```python
from build123d import *

# Parameters (mm, degrees)
BOSS_EXTRUDE1_DEPTH            = 44
CUT_EXTRUDE1_REACH             = 129.516
SKETCH5_R                      = 23
CUT_EXTRUDE1_DIRECTION_2_REACH = 129.516
CUT_EXTRUDE2_REACH             = 137.133
SKETCH6_R                      = 5
CUT_EXTRUDE3_REACH             = 137.133
SKETCH7_R                      = 9.5


with BuildPart() as part:
    # Sketch1 → Boss-Extrude1 (new, symmetric)
    with BuildSketch(Plane(origin=(0, 0, 0), x_dir=(0, 0, -1), z_dir=(1, 0, 0))):
        with BuildLine():
            Line((0, 0), (0, -65))
            Line((0, -65), (12, -65))
            Line((12, -65), (12, -30))
            Line((12, -30), (75, -30))
            Line((75, -30), (75, -27))
            ThreePointArc((75, -27), (75.878679656, -24.878679656), (78, -24))
            Line((78, -24), (110, -24))
            Line((110, -24), (110, 0))
            Line((110, 0), (0, 0))
        make_face()
    extrude(amount=BOSS_EXTRUDE1_DEPTH, both=True)

    # Sketch5 → Cut-Extrude1 (cut, up to next)
    with BuildSketch(Plane(origin=(0, 6.55814551, -14.063988431), x_dir=(1, 0, 0), z_dir=(0, -0.42261826174069383, 0.9063077870366527)), mode=Mode.PRIVATE) as cut_extrude1_sk1:
        with Locations((0, 1.248613111)):
            Circle(SKETCH5_R)
    cut_extrude1_tool1 = extrude(cut_extrude1_sk1.sketch, amount=-CUT_EXTRUDE1_REACH, mode=Mode.PRIVATE) & part.part
    add(cut_extrude1_tool1.solids().sort_by_distance((0, 7.689773, -13.536302))[0], mode=Mode.SUBTRACT)

    # Sketch5 → Cut-Extrude1 direction 2 (cut, up to next)
    with BuildSketch(Plane(origin=(0, 6.55814551, -14.063988431), x_dir=(1, 0, 0), z_dir=(0, -0.42261826174069383, 0.9063077870366527)), mode=Mode.PRIVATE) as cut_extrude1_direction_2_sk1:
        with Locations((0, 1.248613111)):
            Circle(SKETCH5_R)
    cut_extrude1_direction_2_tool1 = extrude(cut_extrude1_direction_2_sk1.sketch, amount=CUT_EXTRUDE1_DIRECTION_2_REACH, mode=Mode.PRIVATE) & part.part
    add(cut_extrude1_direction_2_tool1.solids().sort_by_distance((0, 7.689773, -13.536302))[0], mode=Mode.SUBTRACT)

    # Sketch6 → Cut-Extrude2 (cut, up to next)
    with BuildSketch(Plane(origin=(0, 0, 0), x_dir=(1, 0, 0), z_dir=(0, 1, 0)), mode=Mode.PRIVATE) as cut_extrude2_sk1:
        with Locations(Location((27.5, 95, 0), (0, 0, 270))):
            Circle(SKETCH6_R)
    cut_extrude2_tool1 = extrude(cut_extrude2_sk1.sketch, amount=-CUT_EXTRUDE2_REACH, mode=Mode.PRIVATE) & part.part
    # Sketch6 → Cut-Extrude2 (cut, up to next)
    with BuildSketch(Plane(origin=(0, 0, 0), x_dir=(1, 0, 0), z_dir=(0, 1, 0)), mode=Mode.PRIVATE) as cut_extrude2_sk2:
        with Locations(Location((-27.5, 95, 0), (0, 0, 270))):
            Circle(SKETCH6_R)
    cut_extrude2_tool2 = extrude(cut_extrude2_sk2.sketch, amount=-CUT_EXTRUDE2_REACH, mode=Mode.PRIVATE) & part.part
    # Sketch6 → Cut-Extrude2 (cut, up to next)
    with BuildSketch(Plane(origin=(0, 0, 0), x_dir=(1, 0, 0), z_dir=(0, 1, 0)), mode=Mode.PRIVATE) as cut_extrude2_sk3:
        with Locations(Location((-27.5, 60, 0), (0, 0, 270))):
            Circle(SKETCH6_R)
    cut_extrude2_tool3 = extrude(cut_extrude2_sk3.sketch, amount=-CUT_EXTRUDE2_REACH, mode=Mode.PRIVATE) & part.part
    # Sketch6 → Cut-Extrude2 (cut, up to next)
    with BuildSketch(Plane(origin=(0, 0, 0), x_dir=(1, 0, 0), z_dir=(0, 1, 0)), mode=Mode.PRIVATE) as cut_extrude2_sk4:
        with Locations(Location((27.5, 60, 0), (0, 0, 270))):
            Circle(SKETCH6_R)
    cut_extrude2_tool4 = extrude(cut_extrude2_sk4.sketch, amount=-CUT_EXTRUDE2_REACH, mode=Mode.PRIVATE) & part.part
    add(cut_extrude2_tool1.solids().sort_by_distance((27.5, 0, -95))[0], mode=Mode.SUBTRACT)
    add(cut_extrude2_tool2.solids().sort_by_distance((-27.5, 0, -95))[0], mode=Mode.SUBTRACT)
    add(cut_extrude2_tool3.solids().sort_by_distance((-27.5, 0, -60))[0], mode=Mode.SUBTRACT)
    add(cut_extrude2_tool4.solids().sort_by_distance((27.5, 0, -60))[0], mode=Mode.SUBTRACT)

    # Sketch7 → Cut-Extrude3 (cut, up to next)
    with BuildSketch(Plane.XY, mode=Mode.PRIVATE) as cut_extrude3_sk1:
        with BuildLine():
            Line((44, -65), (44, -24))
            Line((44, -24), (19.769224603, -55.302867659))
            ThreePointArc((19.769224603, -55.302867659), (11.009729981, -62.445174219), (0, -65))
            Line((0, -65), (44, -65))
        make_face()
    cut_extrude3_tool1 = extrude(cut_extrude3_sk1.sketch, amount=-CUT_EXTRUDE3_REACH, mode=Mode.PRIVATE) & part.part
    # Sketch7 → Cut-Extrude3 (cut, up to next)
    with BuildSketch(Plane.XY, mode=Mode.PRIVATE) as cut_extrude3_sk2:
        with Locations((0, -40)):
            Circle(SKETCH7_R)
    cut_extrude3_tool2 = extrude(cut_extrude3_sk2.sketch, amount=-CUT_EXTRUDE3_REACH, mode=Mode.PRIVATE) & part.part
    # Sketch7 → Cut-Extrude3 (cut, up to next)
    with BuildSketch(Plane.XY, mode=Mode.PRIVATE) as cut_extrude3_sk3:
        with BuildLine():
            Line((-44, -65), (0, -65))
            ThreePointArc((0, -65), (-11.009729981, -62.445174219), (-19.769224603, -55.302867659))
            Line((-19.769224603, -55.302867659), (-44, -24))
            Line((-44, -24), (-44, -65))
        make_face()
    cut_extrude3_tool3 = extrude(cut_extrude3_sk3.sketch, amount=-CUT_EXTRUDE3_REACH, mode=Mode.PRIVATE) & part.part
    add(cut_extrude3_tool1.solids().sort_by_distance((32.710915, -51.707074, 0))[0], mode=Mode.SUBTRACT)
    add(cut_extrude3_tool2.solids().sort_by_distance((0, -40, 0))[0], mode=Mode.SUBTRACT)
    add(cut_extrude3_tool3.solids().sort_by_distance((-32.710915, -51.707074, 0))[0], mode=Mode.SUBTRACT)


solid = part.part
```
For this review, take the finished solid that the model builds, in its own axes (mm). A direction names the side the tool comes from. Give positions to 0.01 mm unless a question says otherwise; leave off trailing zeros. Write each loop counter-clockwise with the first axis right and the second up, starting at its lowest first coordinate (ties: lowest second). Pieces come first, ordered by that corner, then holes.
Item 1: Take a section at D-D (x = -4). Give the boundary of the cut face in (y, z), and give its area (3 significant figures).
Item 2: Take a section at A-A (z = -95). Give the boundary of the cut face in (x, y), and give its area (3 significant figures).
Item 3: The part is to be moulded in two halves that separate along Y. For faces 3 (the face through (-1.24, -30.58, -5.92)), 4 (the face through (-39.905, -29.29, -27.262)), 5 (the face through (1, -52, -12)), say which applies: +Y half, -Y half, draft (parallel to the pull), parting line (faces both ways), or undercut.
Item 4: Take a section at C-C (x = 25). Give the boundary of the cut face in (y, z), and give its area (3 significant figures).
Item 5: Insertion check: P1, Ø9, axis at x = 27.5, z = -95, coming from the -Y side; P2, Ø0.9, axis at x = 1.5, y = -29, coming from the -Z side; P3, Ø10, axis at x = -7, z = -71.5, coming from the -Y side; P4, Ø9.5, axis at x = 4, z = -97.5, coming from the -Y side. Each pin has a flat end and moves straight along its axis. Give the tip position at first contact, or say it passes through.
Item 6: Take a section at B-B (y = -32). Give the boundary of the cut face in (x, z), and give its area (3 significant figures).
Item 7: Machinability: for faces 1 (the face through (1, -25, 0)), 2 (the face through (1, -30, -43)), which of the approach directions +Z, -Z, +X, -X, +Y, -Y give a long, thin tool a straight path to every point of the face, cutting with its end or side? Answer none if there is none.
Item 8: Wall thickness on probe 1 along X at (y, z) = (-22.25, -60); probe 2 along Z at (x, y) = (-25.5, -17); probe 3 along Z at (x, y) = (30, -2.5): over which ranges is each line inside the solid? List them lowest first.
Established:
1. outline: (-64.68, -12) - (-48.62, -12) - (-48.62, 0) - (-64.68, 0) - close; (-31.38, -12) - (-30, -12) - (-30, -75) - (-27, -75) arc R3 cw to (-24, -78) - (-24, -110) - (0, -110) - (0, -50.64) - (-23.61, 0) - (-31.38, 0) - close
1. area: 2,700 mm2
2. outline: (-44, -24) - (-32.5, -24) - (-32.5, 0) - (-44, 0) - close; (-22.5, -24) - (22.5, -24) - (22.5, 0) - (-22.5, 0) - close; (32.5, -24) - (44, -24) - (44, 0) - (32.5, 0) - close
2. area: 1,630 mm2
3. face 3: undercut
3. face 4: -Y half
3. face 5: draft
4. outline: (-48.55, -12) - (-30, -12) - (-30, -55.67) - (0, -55.67) - (0, 0) - (-48.55, 0) - close; (-30, -75) - (-27, -75) arc R3 cw to (-24, -78) - (-24, -90.67) - (0, -90.67) - (0, -64.33) - (-30, -64.33) - close; (-24, -110) - (0, -110) - (0, -99.33) - (-24, -99.33) - close
4. area: 2,850 mm2
5. P1: passes through
5. P2: stops at z = -75
5. P3: stops at y = -30
5. P4: stops at y = -24
6. outline: (-37.81, -12) - (-5.12, -12) - (-5.12, 0) - (-37.81, 0) - close; (5.12, -12) - (37.81, -12) - (37.81, 0) - (5.12, 0) - close
6. area: 784 mm2
7. face 1: +Z, +X, -X, +Y, -Y
7. face 2: -Z, +X, -X, -Y
8. probe 1: x = -44 to -32.5, -22.5 to 22.5, 32.5 to 44
8. probe 2: z = -110 to -99.58, -90.42 to -64.58, -55.42 to 0
8. probe 3: z = -110 to -99.33, -90.67 to -64.33, -55.67 to 0
